Work out the finished part from the listing and answer in its coordinate system (mm). Coordinates: 2 decimals unless noted, no trailing zeros. Loops run counter-clockwise (first coordinate to the right, second up) from the corner with the lowest first, then second, coordinate; pieces in that order, holes last. Notation, with made-up numbers: M 37,20.25 L 78,20.25 A25 cw 78,32.25 Z; hole C -11,18.5 d1. An arc over 180 degrees is marked long. Write each question's results on one line, items separated by ' | '.
```python
from build123d import *

# Parameters (mm, degrees)
SKETCH1_R           = 15
BOSS_EXTRUDE1_DEPTH = 15
SKETCH2_R           = 5
CUT_EXTRUDE1_DEPTH  = 15
SKETCH3_R           = 0.595755822
CUT_EXTRUDE2_DEPTH  = 15


with BuildPart() as part:
    # Sketch1 → Boss-Extrude1 (new body)
    with BuildSketch(Plane.XY):
        Circle(SKETCH1_R)
    extrude(amount=BOSS_EXTRUDE1_DEPTH)

    # Sketch2 → Cut-Extrude1 (cut)
    with BuildSketch(Plane.XY.offset(15)):
        Circle(SKETCH2_R)
    extrude(amount=-CUT_EXTRUDE1_DEPTH, mode=Mode.SUBTRACT)

    # Sketch3 → Cut-Extrude2 (cut)
    with BuildSketch(Plane.XY.offset(15)):
        with Locations((0, 15)):
            Circle(SKETCH3_R)
        with Locations((2.087596514, 14.854021031)):
            Circle(SKETCH3_R)
        with Locations((4.134560337, 14.418925439)):
            Circle(SKETCH3_R)
        with Locations((6.101049646, 13.703181865)):
            Circle(SKETCH3_R)
        with Locations((7.948788963, 12.720721442)):
            Circle(SKETCH3_R)
        with Locations((9.641814145, 11.490666647)):
            Circle(SKETCH3_R)
        with Locations((11.147172382, 10.036959095)):
            Circle(SKETCH3_R)
        with Locations((12.435563588, 8.387893552)):
            Circle(SKETCH3_R)
        with Locations((13.481910694, 6.575567202)):
            Circle(SKETCH3_R)
        with Locations((14.265847744, 4.635254916)):
            Circle(SKETCH3_R)
        with Locations((14.772116295, 2.604722665)):
            Circle(SKETCH3_R)
        with Locations((14.990862405, 0.523492451)):
            Circle(SKETCH3_R)
        with Locations((14.917828431, -1.567926949)):
            Circle(SKETCH3_R)
        with Locations((14.554435894, -3.628828434)):
            Circle(SKETCH3_R)
        with Locations((13.907757819, -5.619098901)):
            Circle(SKETCH3_R)
        with Locations((12.990381057, -7.5)):
            Circle(SKETCH3_R)
        with Locations((11.820161304, -9.23492213)):
            Circle(SKETCH3_R)
        with Locations((10.419875557, -10.790097005)):
            Circle(SKETCH3_R)
        with Locations((8.816778784, -12.135254916)):
            Circle(SKETCH3_R)
        with Locations((7.042073442, -13.244213893)):
            Circle(SKETCH3_R)
        with Locations((5.13030215, -14.095389312)):
            Circle(SKETCH3_R)
        with Locations((3.118675362, -14.672214011)):
            Circle(SKETCH3_R)
        with Locations((1.046347106, -14.963460754)):
            Circle(SKETCH3_R)
        with Locations((-1.046347106, -14.963460754)):
            Circle(SKETCH3_R)
        with Locations((-3.118675362, -14.672214011)):
            Circle(SKETCH3_R)
        with Locations((-5.13030215, -14.095389312)):
            Circle(SKETCH3_R)
        with Locations((-7.042073442, -13.244213893)):
            Circle(SKETCH3_R)
        with Locations((-8.816778784, -12.135254916)):
            Circle(SKETCH3_R)
        with Locations((-10.419875557, -10.790097005)):
            Circle(SKETCH3_R)
        with Locations((-11.820161304, -9.23492213)):
            Circle(SKETCH3_R)
        with Locations((-12.990381057, -7.5)):
            Circle(SKETCH3_R)
        with Locations((-13.907757818, -5.619098901)):
            Circle(SKETCH3_R)
        with Locations((-14.554435894, -3.628828434)):
            Circle(SKETCH3_R)
        with Locations((-14.917828431, -1.567926949)):
            Circle(SKETCH3_R)
        with Locations((-14.990862405, 0.523492451)):
            Circle(SKETCH3_R)
        with Locations((-14.772116295, 2.604722665)):
            Circle(SKETCH3_R)
        with Locations((-14.265847744, 4.635254916)):
            Circle(SKETCH3_R)
        with Locations((-13.481910694, 6.575567202)):
            Circle(SKETCH3_R)
        with Locations((-12.435563588, 8.387893552)):
            Circle(SKETCH3_R)
        with Locations((-11.147172382, 10.036959095)):
            Circle(SKETCH3_R)
        with Locations((-9.641814145, 11.490666647)):
            Circle(SKETCH3_R)
        with Locations((-7.948788963, 12.720721442)):
            Circle(SKETCH3_R)
        with Locations((-6.101049646, 13.703181865)):
            Circle(SKETCH3_R)
        with Locations((-4.134560337, 14.418925439)):
            Circle(SKETCH3_R)
        with Locations((-2.087596514, 14.854021031)):
            Circle(SKETCH3_R)
    extrude(amount=-CUT_EXTRUDE2_DEPTH, mode=Mode.SUBTRACT)


solid = part.part
```
1) Given pin 1 Ø10 at (x, y) = (11.5, 11.5) entering from -Z; pin 2 Ø9 at (x, y) = (0, 0) entering from +Z (3 decimals); pin 3 Ø1.5 at (y, z) = (3.5, 8.5) entering from -X; pin 4 Ø8 at (y, z) = (-10.5, 10.5) entering from -X, each flat-ended and moving along its own axis, determine where each tip first touches the part or whether it passes through.
Check result:
pin 1: z = 0 | pin 2: through | pin 3: x = -14.66 | pin 4: x = -13.52
2) Find section C-C, the plane y = -7.5. Give the vertices of the cut face in (x, z).
Check result:
outline: M -12.39,0 L 12.39,0 L 12.39,15 L -12.39,15 Z
3) Find section B-B, the plane y = 1.5. Give the vertices of the cut face in (x, z), and give its area (3 significant figures).
Check result:
outline: M -14.92,0 L -4.77,0 L -4.77,15 L -14.92,15 Z; M 4.77,0 L 14.92,0 L 14.92,15 L 4.77,15 Z | area: 305 mm^2
4) Find section A-A, the plane x = 0. Give the vertices of the cut face in (y, z).
Check result:
outline: M -15,0 L -5,0 L -5,15 L -15,15 Z; M 5,0 L 14.4,0 L 14.4,15 L 5,15 Z
5) For a pull along Y with two mould halves and no side action, classify faces 1 (the face through (-0.013, 14.404, 7.605)), 2 (the face through (14.395, 0.516, 7.605)), 3 (the face through (0, -15, 7)) as released by +Y, released by -Y, zero draft, split by the parting line, or undercut.
Check result:
face 1: released by +Y | face 2: undercut | face 3: released by -Y
6) Straight lines are drawn through the part: probe 1 along Y at (x, z) = (0, 10.5); probe 2 along Y at (x, z) = (8.75, 14); probe 3 along Y at (x, z) = (-3, 5). For each, find the intervals that lie inside material, in ascending order. Write a range as [from, to].
Check result:
probe 1: [-15, -5], [5, 14.4] | probe 2: [-11.54, 12.18] | probe 3: [-14.09, -4], [4, 14.7]
